Study the drawing (mm; zero at the part's minimum x, y, z) and answer. A direction names the side the tool comes from. Give positions to 0.01 mm unless a question says otherwise; leave off trailing zeros. Write each loop counter-clockwise with the first axis right and the second up, starting at its lowest first coordinate (ties: lowest second). Pieces come first, ordered by that corner, then holes.
1) Find section B-B (y = 18.5). Determine the outline of the cut face in (x, z).
2) Find section C-C (z = 10). Determine the outline of the cut face in (x, y), plus the area to 3 significant figures.
3) Find section D-D (x = 38). Determine the outline of the cut face in (y, z).
4) A tool of negligible diameter and unlimited length cuts with its end or side. For the marked faces 1, 2 and 3, from which of +Z, -Z, +X, -X, +Y, -Y can it reach the whole face along a straight path? Write none if from no direction.
5) Straight lines are drawn through the part: probe 1 along X at (y, z) = (4, 10.25); probe 2 along Y at (x, z) = (35, 12.5); probe 3 along Y at (x, z) = (11, 17.5). For each, find the intervals that lie inside material, in ascending order.
6) Find section A-A (x = 51). Determine the outline of the cut face in (y, z), plus the area to 3 significant figures.
7) Given pin 1 Ø4 at (x, z) = (33, 16.5) entering from +Y; pin 2 Ø4.5 at (x, z) = (42, 9.5) entering from +Y; pin 3 Ø1 at (x, y) = (39.5, 37.5) entering from +Z, each flat-ended and moving along its own axis, determine where each tip first touches the part or whether it passes through.
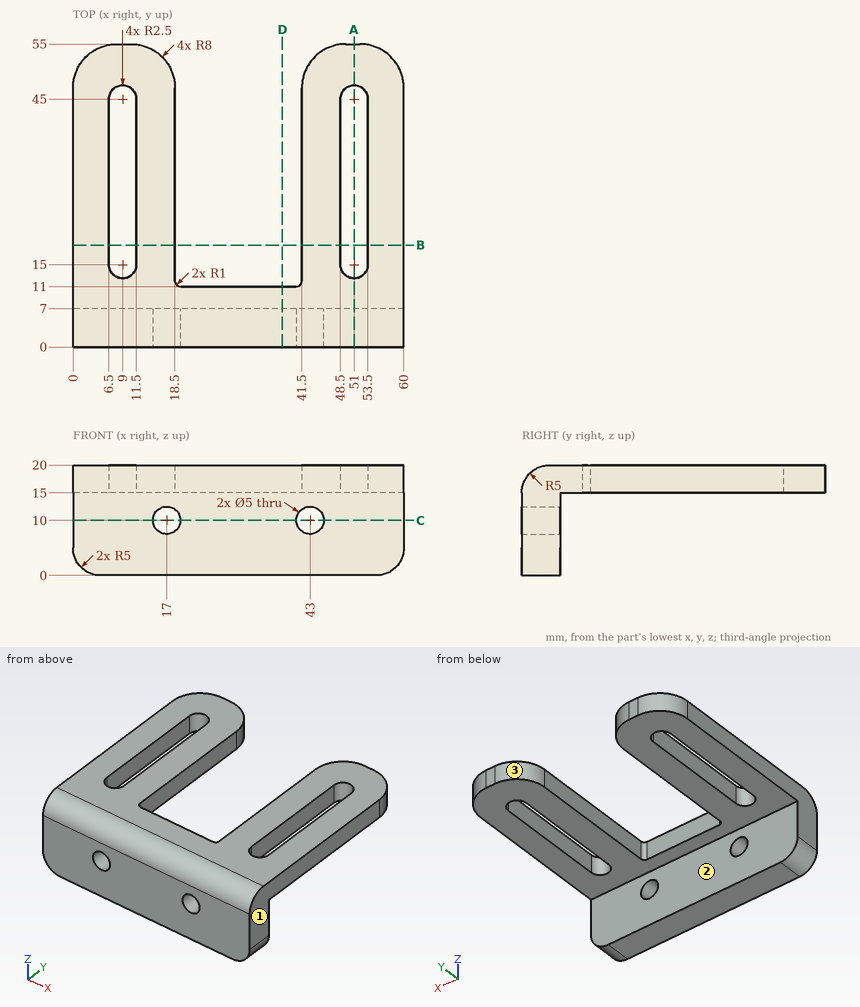
Results:
1. outline: (0, 15) - (6.5, 15) - (6.5, 20) - (0, 20) - close; (11.5, 15) - (18.5, 15) - (18.5, 20) - (11.5, 20) - close; (41.5, 15) - (48.5, 15) - (48.5, 20) - (41.5, 20) - close; (53.5, 15) - (60, 15) - (60, 20) - (53.5, 20) - close
2. outline: (0, 0) - (14.5, 0) - (14.5, 7) - (0, 7) - close; (19.5, 0) - (40.5, 0) - (40.5, 7) - (19.5, 7) - close; (45.5, 0) - (60, 0) - (60, 7) - (45.5, 7) - close
2. area: 350 mm2
3. outline: (0, 0) - (7, 0) - (7, 15) - (11, 15) - (11, 20) - (5, 20) arc R5 ccw to (0, 15) - close
4. face 1: +Z, -Z, +X, +Y, -Y
4. face 2: -Z, +X, -X, +Y
4. face 3: +Z, -Z, +Y
5. probe 1: x = 0 to 14.51, 19.49 to 40.51, 45.49 to 60
5. probe 2: y = 0 to 7
5. probe 3: y = 0.67 to 13.5, 46.5 to 54.98
6. outline: (0, 0) - (7, 0) - (7, 15) - (12.5, 15) - (12.5, 20) - (5, 20) arc R5 ccw to (0, 15) - close; (47.5, 15) - (55, 15) - (55, 20) - (47.5, 20) - close
6. area: 200 mm2
7. pin 1: stops at y = 11
7. pin 2: stops at y = 7
7. pin 3: passes through
